Can you work these out from the model? Positions are in its coordinate system, mm. Face numbers are marked on the shaded views. A direction names the side the tool comes from. Give positions to 0.01 mm unless a question says otherwise; leave off trailing zeros. Loops run counter-clockwise (first coordinate to the right, second up) from the corner with the lowest first, then second, coordinate; pieces in that order, holes last. Notation, with made-up numbers: M 58,-0.75 L 108,-0.75 A36 cw 108,35.25 Z; hole C 77.5,-30 d2. An arc over 180 degrees is marked long. One line per item, written item: value. Start each with the question number.
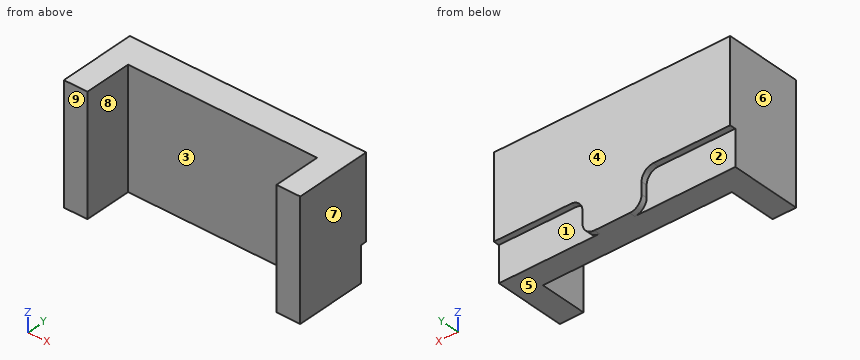
from build123d import *

# Parameters (mm, degrees)
BOSS_EXTRUDE1_DEPTH = 100
SKETCH2_W           = 50
SKETCH2_H           = 30
BOSS_EXTRUDE2_DEPTH = 5
FILLET1_R           = 10
SCALE1_SCALE        = 10


with BuildPart() as part:
    # Sketch1 → Boss-Extrude1 (new body)
    with BuildSketch(Plane.XY):
        Polygon((0, 60), (-100, 60), (-100, 0), (-80, 0), (-80, 40), (0, 40), align=None)
    boss_extrude1 = extrude(amount=BOSS_EXTRUDE1_DEPTH)

    # Mirror1: Boss-Extrude1 across plane
    add(boss_extrude1.mirror(Plane(origin=(0, 40, 100), x_dir=(0, 0, 1), z_dir=(-1, 0, 0))))

    # Sketch2 → Boss-Extrude2 (add)
    with BuildSketch(Plane(origin=(0, 60, 0), x_dir=(1, 0, 0), z_dir=(0, 1, 0))):
        Polygon((-100, -30), (-100, -100), (100, -100), (100, -30), (25, -30), (-25, -30), align=None)
        with Locations((0, -15)):
            Rectangle(SKETCH2_W, SKETCH2_H)
    extrude(amount=BOSS_EXTRUDE2_DEPTH)

    # Fillet1
    fillet1_edges = [part.edges().sort_by_distance(p)[0] for p in [
        (-25, 62.5, 30),
        (25, 62.5, 30),
        (25, 62.5, 0),
        (-25, 62.5, 0),
    ]]
    fillet(fillet1_edges, radius=FILLET1_R)


with BuildPart() as part_1:
    # Scale1: scaled about (0, 43.990196078, 51.243889179)
    add(part.part.scale(SCALE1_SCALE).moved(Location((0, -395.911764702, -461.195002611))))


solid = part_1.part
Q1. If we section it at D-D, the plane x = -181: Write out the boundary of the cut face in (y, z) (3 decimals).
Q2. Which directions (+Z, -Z, +X, -X, +Y, -Y) give clear straight access to the entire face, cutting with the end or side of a thin tool? Please do the marked faces 1, 2, 3, 4 and 5.
Q3. If we section it at C-C, the plane x = 752.5: Write out the boundary of the cut face in (y, z) (3 decimals).
Q4. For P1, Ø25, axis at y = 241.5, z = -298, coming from the +X side; P2, Ø4, axis at x = -498, z = -177.5, coming from the +Y side; P3, Ø15, axis at x = 706, y = 237, coming from the -Z side (3 decimals), each with a flat end and sliding along its axis, tell me the tip position at first contact or that it passes through.
Q5. I need wall thicknesses on line 1 along X through (y, z) = (-157, 211); line 2 along Y through (x, z) = (-788, -33); line 3 along Z through (x, y) = (662, 225) (3 decimals). Which ranges of each line are inside material? Lowest first, please.
Q6. If we mould it in two halves opening along X, with no side actions, what happens to the marked faces 6, 7, 8 and 9? For each: released by +X, released by -X, zero draft, split by the parting line, or undercut.
Q7. If we section it at A-A, the plane y = -318: Write out the boundary of the cut face in (x, z) (3 decimals), plus the area to 3 significant figures.
Q8. If we section it at B-B, the plane z = 169.5: Write out the boundary of the cut face in (x, y), plus the area to 3 significant figures.
Response:
1. outline: M 4.088,-461.195 L 204.088,-461.195 L 204.088,-456.269 L 254.088,-456.269 L 254.088,538.805 L 4.088,538.805 Z
2. face 1: -Z, +X, +Y
2. face 2: -Z, -X, +Y
2. face 3: +Z, -Z, -Y
2. face 4: +Z, -Z, +X, -X, +Y
2. face 5: -Z, +X, -X, +Y, -Y
3. outline: M 4.088,-461.195 L 204.088,-461.195 L 204.088,-161.195 L 254.088,-161.195 L 254.088,538.805 L 4.088,538.805 Z
4. P1: x = 250
4. P2: y = 204.09
4. P3: z = -161.195
5. line 1: -1000 to -800, 800 to 1000
5. line 2: 4.09 to 254.09
5. line 3: -161.195 to 538.805
6. face 6: released by -X
6. face 7: released by +X
6. face 8: undercut
6. face 9: zero draft
7. outline: M -1000,-461.195 L -800,-461.195 L -800,538.805 L -1000,538.805 Z; M 800,-461.195 L 1000,-461.195 L 1000,538.805 L 800,538.805 Z
7. area: 400,000 mm^2
8. outline: M -1000,-395.91 L -800,-395.91 L -800,4.09 L 800,4.09 L 800,-395.91 L 1000,-395.91 L 1000,254.09 L -1000,254.09 Z
8. area: 660,000 mm^2
